The model under review builds one solid part; all positions refer to its coordinate system, in mm. A direction names the side the tool comes from. Coordinates: 2 decimals unless noted, no trailing zeros. Order: outer loops, then holes, each group sorted by start corner. A loop starts at its lowest first (then second) coordinate and runs counter-clockwise, first axis right, second up. Notation, with made-up numbers: (16.25, 11.5) -> (60.25, 11.5) arc R17 cw to (60.25, 33.5) -> close; hole circle Ø4 at (29, 67.25). An arc over 180 degrees is marked (long way). Put each result on its own line as item: value.
from build123d import *

# Parameters (mm, degrees)
F0_R     = 22.225
F1_DEPTH = 1.5875
F2_R     = 0.79375
F3_R     = 22.225
F3_R_2   = 7.9375
F4_DEPTH = 0.762


with BuildPart() as f1:
    # F0 (on Front) → F1 (new body)
    with BuildSketch(Plane.XZ):
        Circle(F0_R)
    extrude(amount=F1_DEPTH)

    # F2
    f2_edges = [f1.edges().sort_by_distance(p)[0] for p in [
        (-22.225, -1.5875, 0),
    ]]
    fillet(f2_edges, radius=F2_R)

    # F3 (on face) → F4 (join)
    with BuildSketch(Plane(origin=(0, 0, 0), x_dir=(-1, 0, 0), z_dir=(0, 1, 0))):
        Circle(F3_R)
        Circle(F3_R_2, mode=Mode.SUBTRACT)
    extrude(amount=F4_DEPTH)


solid = f1.part
Item 1: For line 1 (Z direction, x = 0, y = 0.25) (1 decimal); line 2 (Z direction, x = -0.5, y = -0.5); line 3 (X direction, y = 0.4, z = -4), list the stretches that pass through material, from the lowest coordinate up. Write a range as from..to.
Answers below:
line 1: -22.2..-7.9, 7.9..22.2
line 2: -22.22..22.22
line 3: -21.86..-6.86, 6.86..21.86
Item 2: For faces 3 (the cylindrical face through (1.72, 0.38, -7.75)), 4 (the flat face through (0, -1.588, 0)), list the 3-axis set-ups (+Z, -Z, +X, -X, +Y, -Y) from which the entire face can be reached by the end or side of a thin tool; tool diameter is ignored.
Answers below:
face 3: +Y
face 4: +Z, -Z, +X, -X, -Y
Item 3: Mouldability with a two-part tool opening along Z and no side actions: class faces 1 (the flat face through (0, 0.762, -10)), 2 (the flat face through (0, 0, 0)) as +Z half, -Z half, draft (parallel to the pull), parting line (faces both ways), or undercut.
Answers below:
face 1: draft
face 2: undercut
Item 4: Consider section A-A on z = 0. Write out the cut boundary in (x, y) (1 decimal).
Answers below:
outline: (-22.2, -0.8) arc R0.8 ccw to (-21.4, -1.6) -> (21.4, -1.6) arc R0.8 ccw to (22.2, -0.8) -> (22.2, 0.8) -> (7.9, 0.8) -> (7.9, 0) -> (-7.9, 0) -> (-7.9, 0.8) -> (-22.2, 0.8) -> close
Item 5: Consider section B-B on x = 0. Write out the cut boundary in (y, z) (1 decimal), and give its area (3 significant figures).
Answers below:
outline: (-1.6, -21.4) arc R0.8 ccw to (-0.8, -22.2) -> (0.8, -22.2) -> (0.8, -7.9) -> (0, -7.9) -> (0, 7.9) -> (0.8, 7.9) -> (0.8, 22.2) -> (-0.8, 22.2) arc R0.8 ccw to (-1.6, 21.4) -> close
area: 92.1 mm^2
Item 6: For pin 1 Ø5 at (x, z) = (0.5, 0) entering from +Y, flat-tipped, find the tip position at first contact; note if it passes through.
Answers below:
pin 1: y = 0
